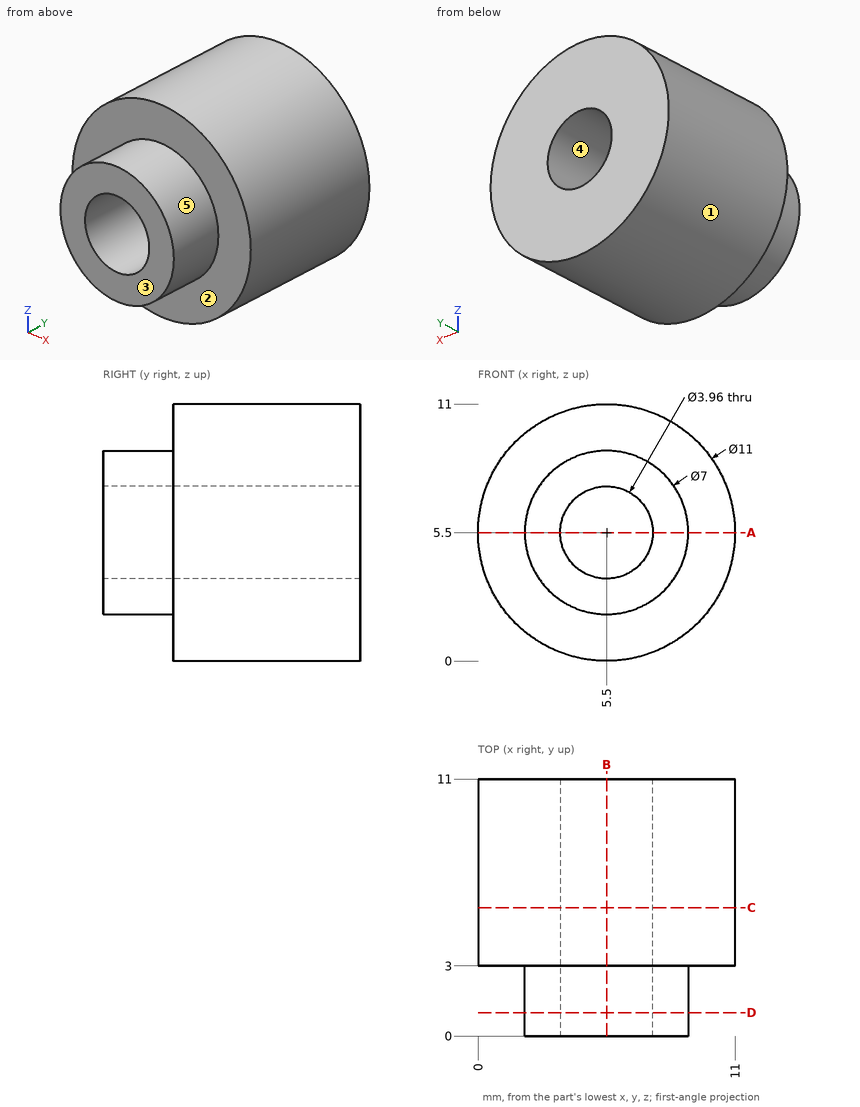
Print and shaded views of the part. All mm, measured from the part's lowest x, y and z. A direction names the side the tool comes from. Coordinates: 2 decimals unless noted, no trailing zeros. Loops run counter-clockwise (first coordinate to the right, second up) from the corner with the lowest first, then second, coordinate; pieces in that order, holes last. Notation, with made-up numbers: (-4, -13.75) - (9, -13.75) arc R36 cw to (9, 20.25) - close; hole circle Ø2 at (22.25, 28). An arc over 180 degrees is marked (long way). Use one line per item in the form item = value. Start each with the question number.
1) Band-saw the part on D-D (y = 1). Give the cut face in (x, z).
2) Band-saw the part on A-A (z = 5.5). Give the cut face in (x, y), and give its area (3 significant figures).
3) Two-plate mould, pull along X, no slides. Class the marked faces 3, 4 and 5: +X half, -X half, draft (parallel to the pull), parting line (faces both ways), or undercut.
4) Band-saw the part on B-B (x = 5.5). Give the cut face in (y, z).
5) Flat gauge pins, fed straight in: pin 1 (1 mm diameter, centred on y = 10, z = 3, fed in from -X); pin 2 (5 mm diameter, centred on y = 3, z = 1.5, fed in from +X); pin 3 (1 mm diameter, centred on x = 9.5, z = 3, fed in from -Y). Where does each tip first touch, or does it go through?
6) Tool access for the marked faces 1 and 2: list every direction of +Z, -Z, +X, -X, +Y, -Y with a clear straight run to the whole face (end or side of a thin tool).
7) Band-saw the part on C-C (y = 5.5). Give the cut face in (x, z).
8) Drill centre lines: L1, parallel to X at y = 6, z = 5.5; L2, parallel to Y at x = 9, z = 3; L3, parallel to Z at x = 6.75, y = 10.25. Where is each one in solid material? Low to high. Write a range as from..to.
Check values:
q1.outline = circle Ø7 at (5.5, 5.5); hole circle Ø3.96 at (5.5, 5.5)
q2.outline = (0, 3) - (2, 3) - (2, 0) - (3.52, 0) - (3.52, 11) - (0, 11) - close; (7.48, 0) - (9, 0) - (9, 3) - (11, 3) - (11, 11) - (7.48, 11) - close
q2.area = 65.4 mm2
q3.face_3 = draft
q3.face_4 = undercut
q3.face_5 = parting line
q4.outline = (0, 2) - (3, 2) - (3, 0) - (11, 0) - (11, 3.52) - (0, 3.52) - close; (0, 7.48) - (11, 7.48) - (11, 11) - (3, 11) - (3, 9) - (0, 9) - close
q5.pin_1 = 0.38
q5.pin_2 = 10.79
q5.pin_3 = 3
q6.face_1 = +Y, -Y
q6.face_2 = -Y
q7.outline = circle Ø11 at (5.5, 5.5); hole circle Ø3.96 at (5.5, 5.5)
q8.L1 = 0..3.52, 7.48..11
q8.L2 = 3..11
q8.L3 = 0.14..3.96, 7.04..10.86
